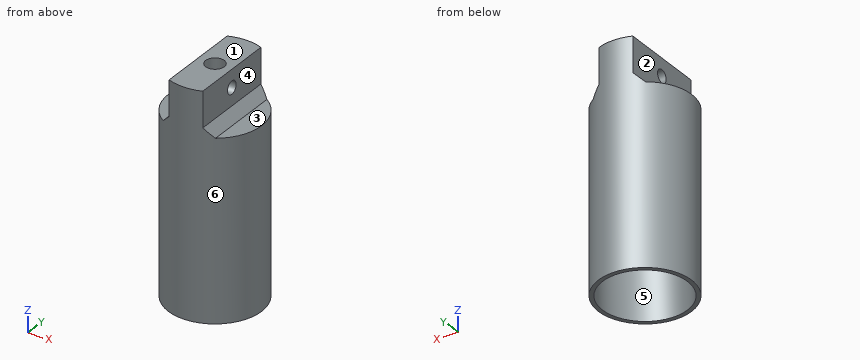
```python
from build123d import *

# Parameters (mm, degrees)
F0_R      = 7.95
F1_DEPTH  = 38.1
F2_R      = 7.2485
F3_DEPTH  = 9.525
F4_R      = 4.7625
F5_DEPTH  = 15.24
F6_R      = 1.6
F7_DEPTH  = 25.4
F8_W      = 5.08
F8_H      = 14.827758
F9_DEPTH  = 7.62
F10_R     = 1.1
F11_DEPTH = 25.4
F12_SIZE  = 1.6


with BuildPart() as f1:
    # F0 (on Top) → F1 (new body)
    with BuildSketch(Plane.XY):
        Circle(F0_R)
    extrude(amount=F1_DEPTH)

    # F2 (on face) → F3 (cut)
    with BuildSketch(Plane(origin=(0, 0, 0), x_dir=(1, 0, 0), z_dir=(0, 0, -1))):
        Circle(F2_R)
    extrude(amount=-F3_DEPTH, mode=Mode.SUBTRACT)

    # F4 (on face) → F5 (cut)
    with BuildSketch(Plane(origin=(0, 0, 9.525), x_dir=(1, 0, 0), z_dir=(0, 0, -1))):
        Circle(F4_R)
    extrude(amount=-F5_DEPTH, mode=Mode.SUBTRACT)

    # F6 (on face) → F7 (cut)
    with BuildSketch(Plane.XY.offset(38.1)):
        Circle(F6_R)
    extrude(amount=-F7_DEPTH, mode=Mode.SUBTRACT)

    # F8 (on face) → F9 (cut)
    with BuildSketch(Plane.XY.offset(38.1)):
        with Locations((-5.41, 0)):
            Rectangle(F8_W, F8_H)
        with Locations((5.41, 0)):
            Rectangle(F8_W, F8_H)
    extrude(amount=-F9_DEPTH, mode=Mode.SUBTRACT)

    # F10 (on face) → F11 (cut)
    with BuildSketch(Plane(origin=(-2.87, 0, 0), x_dir=(0, -1, 0), z_dir=(-1, 0, 0))):
        with Locations((0, 35.1)):
            Circle(F10_R)
    extrude(amount=-F11_DEPTH, mode=Mode.SUBTRACT)

    # F12
    f12_edges = [f1.edges().sort_by_distance(p)[0] for p in [
        (-2.87, 0, 30.48),
        (2.87, 0, 30.48),
    ]]
    chamfer(f12_edges, length=F12_SIZE)


solid = f1.part
```
The model under review builds one solid part; all positions refer to its coordinate system, in mm. Face numbers are marked on the shaded views. A direction names the side the tool comes from. Round coordinates to 2 decimals unless told otherwise and drop trailing zeros. Order: outer loops, then holes, each group sorted by start corner. A loop starts at its lowest first (then second) coordinate and runs counter-clockwise, first axis right, second up.
Item 1: Add section B-B, the plane z = 35.1. State the section outline as (x, y) points, and give its area (3 significant figures).
Working result:
outline: (-2.87, -7.41) arc R7.95 ccw to (2.87, -7.41) - (2.87, -1.1) - (1.16, -1.1) arc R1.6 cw to (-1.16, -1.1) - (-2.87, -1.1) - close; (-2.87, 1.1) - (-1.16, 1.1) arc R1.6 cw to (1.16, 1.1) - (2.87, 1.1) - (2.87, 7.41) arc R7.95 ccw to (-2.87, 7.41) - close
area: 75.0 mm2
Item 2: Draft analysis for pull direction Y (two halves, no side actions). For the marked faces 4, 5 and 6, state which applies: released by +Y, released by -Y, zero draft, split by the parting line, or undercut.
Working result:
face 4: zero draft
face 5: undercut
face 6: split by the parting line
Item 3: For pin 1 (2 mm diameter, centred on y = -4.5, z = 28.5, fed in from -X); pin 2 (3.5 mm diameter, centred on y = 0, z = 35.1, fed in from +X); pin 3 (5.5 mm diameter, centred on x = 0, y = 0, fed in from -Z) (3 decimals), all flat-tipped, find the tip position at first contact; note any pin that passes through.
Working result:
pin 1: stops at x = -7.14
pin 2: stops at x = 2.87
pin 3: stops at z = 24.765
Item 4: Add section C-C, the plane y = 0. Count the separate pieces of the cut face and the enclosed holes in it, and give its area (3 significant figures).
Working result:
separate pieces: 4
enclosed holes: 0
area: 199 mm2
Item 5: To check wall thickness, follow probe 1 along Y at (x, z) = (0, 29.5); probe 2 along Y at (x, z) = (0, 3). State the ranges of each line that lie inside material, in increasing order.
Working result:
probe 1: y = -7.95 to -1.6, 1.6 to 7.95
probe 2: y = -7.95 to -7.25, 7.25 to 7.95
Item 6: Machinability: for the marked faces 1, 2 and 3, which of the approach directions +Z, -Z, +X, -X, +Y, -Y give a long, thin tool a straight path to every point of the face, cutting with its end or side? Answer none if there is none.
Working result:
face 1: +Z, +X, -X, +Y, -Y
face 2: +Z, -X, +Y, -Y
face 3: +Z, +X, +Y, -Y
